```python
from build123d import *

# Parameters (mm, degrees)
SKETCH_1_R          = 3
EXTRUDE_1_DEPTH     = 20
SKETCH_2_W          = 31.985989971
SKETCH_2_H          = 30
CUT_EXTRUDE_2_DEPTH = 64.639610307
SKETCH_3_W          = 45
SKETCH_3_H          = 30
CUT_EXTRUDE_3_DEPTH = 64.639610307


with BuildPart() as part:
    # 草图1 → 凸台-拉伸1 (new body)
    with BuildSketch(Plane.XY):
        with BuildLine():
            Line((-45, 15), (45, 15))
            Line((45, 15), (45, -15))
            Line((45, -15), (-45, -15))
            ThreePointArc((-45, -15), (-60, 0), (-45, 15))
        make_face()
        with Locations((-45, 0)):
            Circle(SKETCH_1_R, mode=Mode.SUBTRACT)
    extrude(amount=EXTRUDE_1_DEPTH)

    # 草图2 → 切除-拉伸2 (cut, through all)
    with BuildSketch(Plane.XY.offset(15)):
        with Locations((-45.637141889, 0)):
            Rectangle(SKETCH_2_W, SKETCH_2_H)
    extrude(amount=-CUT_EXTRUDE_2_DEPTH, mode=Mode.SUBTRACT)

    # 草图3 → 切除-拉伸3 (cut, through all)
    with BuildSketch(Plane.XY.offset(15)):
        with Locations((-37.384024781, 0)):
            Rectangle(SKETCH_3_W, SKETCH_3_H)
    extrude(amount=-CUT_EXTRUDE_3_DEPTH, mode=Mode.SUBTRACT)


solid = part.part
```
Source: CAD feature listing. Evaluate the final solid. Frame: model axes, mm. A direction names the side the tool comes from. Round coordinates to 2 decimals unless told otherwise and drop trailing zeros. Loops run counter-clockwise (first coordinate to the right, second up) from the corner with the lowest first, then second, coordinate; pieces in that order, holes last.
(1) Section query B-B (z = 16.25). Output: boundary loops of the cut face in (x, y), and give its area (3 significant figures).
From the geometry:
outline: (-45, -15) - (45, -15) - (45, 15) - (-45, 15) arc R15 ccw to start; hole circle Ø6 at (-45, 0)
area: 3,030 mm2
(2) Contact query for flat-ended pins moving along their axis: pin 1 Ø8 at (x, y) = (-45, 0) entering from -Z; pin 2 Ø3 at (y, z) = (-3.5, 9) entering from -X; pin 3 Ø8 at (y, z) = (-8.5, 12) entering from -X. Output: stop coordinate, or through.
From the geometry:
pin 1: stops at z = 15
pin 2: stops at x = -14.88
pin 3: stops at x = -58.81
(3) Access query for faces 1 (the flat face through (-38, 0, 15)), 2 (the flat face through (-7, 0, 20)). Directions: +Z, -Z, +X, -X, +Y, -Y. A direction counts if a zero-diameter tool reaches every point of the face in a straight line with its end or side. Return the directions, or none.
From the geometry:
face 1: -Z, -X, +Y, -Y
face 2: +Z, +X, -X, +Y, -Y
(4) Material intervals for probe 1 along X at (y, z) = (0, 17.95); probe 2 along Y at (x, z) = (-45, 18.9); probe 3 along Z at (x, y) = (-15.5, -12.25), sorted ascending.
From the geometry:
probe 1: x = -60 to -48, -42 to 45
probe 2: y = -15 to -3, 3 to 15
probe 3: z = 15 to 20
(5) Section query A-A (y = 0). Output: boundary loops of the cut face in (x, z).
From the geometry:
outline: (-60, 15) - (-48, 15) - (-48, 20) - (-60, 20) - close; (-42, 15) - (-14.88, 15) - (-14.88, 0) - (45, 0) - (45, 20) - (-42, 20) - close
(6) Section query C-C (x = -30.5). Output: boundary loops of the cut face in (y, z), and give its area (3 significant figures).
From the geometry:
outline: (-15, 15) - (15, 15) - (15, 20) - (-15, 20) - close
area: 150 mm2
(7) Section query D-D (z = 4). Output: boundary loops of the cut face in (x, y), and give its area (3 significant figures).
From the geometry:
outline: (-14.88, -15) - (45, -15) - (45, 15) - (-14.88, 15) - close
area: 1,800 mm2
